The listing builds one solid part. Answer for the finished solid, in the listing's coordinates (mm). Face numbers are marked on the shaded views. A direction names the side the tool comes from. Round coordinates to 2 decimals unless told otherwise and drop trailing zeros. Write each loop counter-clockwise with the first axis right and the second up, starting at its lowest first coordinate (ties: lowest second). Pieces come first, ordered by that corner, then holes. Notation, with made-up numbers: (-2.75, 22) - (4.25, 22) arc R30 ccw to (4.25, 52) - close; hole circle Ø3 at (11.25, 66.25). An arc over 180 degrees is marked (long way). Answer in a Markdown table with one row per item.
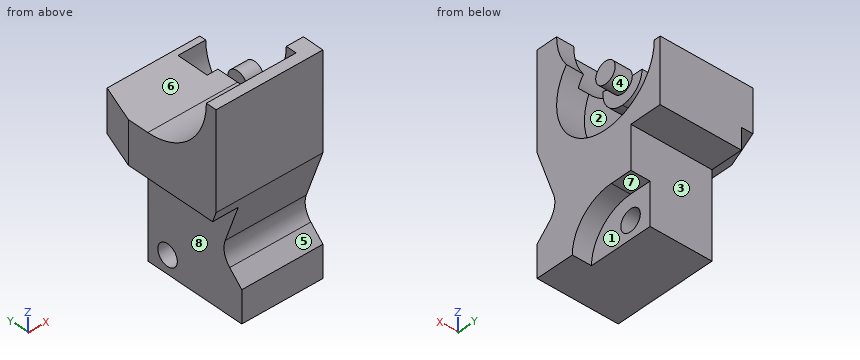
from build123d import *

# Parameters (mm, degrees)
SKETCH1_W           = 100
SKETCH1_H           = 63
BOSS_EXTRUDE1_DEPTH = 50
SKETCH2_W           = 50
SKETCH2_H           = 40
CUT_EXTRUDE1_DEPTH  = 15
SKETCH3_W           = 12
SKETCH3_H           = 10
CUT_EXTRUDE2_DEPTH  = 15
CUT_EXTRUDE3_DEPTH  = 9
SKETCH5_R           = 5
CUT_EXTRUDE4_DEPTH  = 42
CUT_EXTRUDE5_DEPTH  = 51
CUT_EXTRUDE6_DEPTH  = 42
CUT_EXTRUDE10_DEPTH = 51
CUT_EXTRUDE16_DEPTH = 13
CUT_EXTRUDE17_DEPTH = 8
SKETCH11_10_R       = 5
BOSS_EXTRUDE5_DEPTH = 8
CUT_EXTRUDE18_DEPTH = 20
CUT_EXTRUDE22_DEPTH = 8
SKETCH16_W          = 12
SKETCH16_H          = 50
CUT_EXTRUDE23_DEPTH = 49


with BuildPart() as part:
    # Sketch1 → Boss-Extrude1 (new body)
    with BuildSketch(Plane(origin=(0, 0, 0), x_dir=(0, 0, -1), z_dir=(1, 0, 0))):
        with Locations((6.649757701, 6.248490946)):
            Rectangle(SKETCH1_W, SKETCH1_H)
    extrude(amount=-BOSS_EXTRUDE1_DEPTH)

    # Sketch2 → Cut-Extrude1 (cut)
    with BuildSketch(Plane(origin=(0, 37.748490946, 0), x_dir=(1, 0, 0), z_dir=(0, 1, 0))):
        with Locations((-25, 36.649757701)):
            Rectangle(SKETCH2_W, SKETCH2_H)
    extrude(amount=-CUT_EXTRUDE1_DEPTH, mode=Mode.SUBTRACT)

    # Sketch3 → Cut-Extrude2 (cut)
    with BuildSketch(Plane(origin=(0, 37.748490946, 0), x_dir=(1, 0, 0), z_dir=(0, 1, 0))):
        with Locations((-44, 11.649757701)):
            Rectangle(SKETCH3_W, SKETCH3_H)
    extrude(amount=-CUT_EXTRUDE2_DEPTH, mode=Mode.SUBTRACT)

    # Sketch4 → Cut-Extrude3 (cut)
    with BuildSketch(Plane(origin=(0, 0, 0), x_dir=(0, 0, -1), z_dir=(1, 0, 0))):
        with BuildLine():
            Line((36.814050896, 22.748490946), (36.814050896, 12.748490946))
            ThreePointArc((36.814050896, 12.748490946), (42.613947659, -1.335438479), (56.649757701, -7.250834237))
            Line((56.649757701, -7.250834237), (56.649757701, 22.748490946))
            Line((56.649757701, 22.748490946), (36.814050896, 22.748490946))
        make_face()
    extrude(amount=-CUT_EXTRUDE3_DEPTH, mode=Mode.SUBTRACT)

    # Sketch5 → Cut-Extrude4 (cut, through all)
    with BuildSketch(Plane(origin=(-9, 0, 0), x_dir=(0, 0, -1), z_dir=(1, 0, 0))):
        with Locations((48.259112346, 12.748490946)):
            Circle(SKETCH5_R)
    extrude(amount=-CUT_EXTRUDE4_DEPTH, mode=Mode.SUBTRACT)

    # Sketch6 → Cut-Extrude5 (cut, through all)
    with BuildSketch(Plane(origin=(0, 0, 0), x_dir=(0, 0, -1), z_dir=(1, 0, 0))):
        with BuildLine():
            Line((41.649757701, -25.251509054), (35.480677879, -19.082429233))
            ThreePointArc((35.480677879, -19.082429233), (30.574006207, -16.390536973), (24.989408634, -16.756570837))
            Line((24.989408634, -16.756570837), (1.649757701, -25.251509054))
            Line((1.649757701, -25.251509054), (41.649757701, -25.251509054))
        make_face()
    extrude(amount=-CUT_EXTRUDE5_DEPTH, mode=Mode.SUBTRACT)

    # Sketch8 → Cut-Extrude6 (cut)
    with BuildSketch(Plane.ZY.offset(50)):
        with BuildLine():
            Line((43.350242299, -20.251509054), (43.350242299, 9.748490946))
            Line((43.350242299, 9.748490946), (13.350242299, 9.748490946))
            ThreePointArc((13.350242299, 9.748490946), (22.137038863, -11.46471249), (43.350242299, -20.251509054))
        make_face()
    extrude(amount=-CUT_EXTRUDE6_DEPTH, mode=Mode.SUBTRACT)

    # Sketch8<5> → Cut-Extrude10 (cut, through all)
    with BuildSketch(Plane.ZY.offset(50)):
        Polygon((13.350242299, 9.748490946), (43.350242299, 9.748490946), (43.350242299, 37.748490946), (36.798778082, 37.748490946), (13.350242299, 37.748490946), align=None)
    extrude(amount=-CUT_EXTRUDE10_DEPTH, mode=Mode.SUBTRACT)

    # Sketch11 → Cut-Extrude16 (cut)
    with BuildSketch(Plane(origin=(0, 0, 0), x_dir=(0, 0, -1), z_dir=(1, 0, 0))):
        with BuildLine():
            ThreePointArc((-23.350242299, 9.748490946), (-20.421310111, 16.819558758), (-13.350242299, 19.748490946))
            Line((-13.350242299, 19.748490946), (-13.350242299, 34.748490946))
            ThreePointArc((-13.350242299, 34.748490946), (-31.027911829, 27.426160475), (-38.350242299, 9.748490946))
            Line((-38.350242299, 9.748490946), (-23.350242299, 9.748490946))
        make_face()
        with BuildLine():
            Line((-13.350242299, 34.748490946), (-13.350242299, 19.748490946))
            ThreePointArc((-13.350242299, 19.748490946), (-6.279174487, 16.819558758), (-3.350242299, 9.748490946))
            ThreePointArc((-3.350242299, 9.748490946), (-13.350242299, -0.251509054), (-23.350242299, 9.748490946))
            Line((-23.350242299, 9.748490946), (-38.350242299, 9.748490946))
            ThreePointArc((-38.350242299, 9.748490946), (-35.710922074, -1.431848942), (-28.350242299, -10.251509054))
            ThreePointArc((-28.350242299, -10.251509054), (-2.169902411, -12.612188829), (11.649757701, 9.748490946))
            ThreePointArc((11.649757701, 9.748490946), (4.327427231, 27.426160475), (-13.350242299, 34.748490946))
        make_face()
    extrude(amount=-CUT_EXTRUDE16_DEPTH, mode=Mode.SUBTRACT)

    # Sketch11<8> → Cut-Extrude17 (cut)
    with BuildSketch(Plane(origin=(0, 0, 0), x_dir=(0, 0, -1), z_dir=(1, 0, 0))):
        with BuildLine():
            ThreePointArc((-3.350242299, 9.748490946), (-6.279174487, 16.819558758), (-13.350242299, 19.748490946))
            Line((-13.350242299, 19.748490946), (-13.350242299, 14.748490946))
            ThreePointArc((-13.350242299, 14.748490946), (-9.814708393, 13.284024852), (-8.350242299, 9.748490946))
            ThreePointArc((-8.350242299, 9.748490946), (-13.350242299, 4.748490946), (-18.350242299, 9.748490946))
            Line((-18.350242299, 9.748490946), (-23.350242299, 9.748490946))
            ThreePointArc((-23.350242299, 9.748490946), (-13.350242299, -0.251509054), (-3.350242299, 9.748490946))
        make_face()
    extrude(amount=-CUT_EXTRUDE17_DEPTH, mode=Mode.SUBTRACT)

    # Sketch11<10> → Boss-Extrude5 (add)
    with BuildSketch(Plane(origin=(0, 0, 0), x_dir=(0, 0, -1), z_dir=(1, 0, 0))):
        with Locations((-13.350242299, 9.748490946)):
            Circle(SKETCH11_10_R)
    extrude(amount=-BOSS_EXTRUDE5_DEPTH)

    # Sketch14 → Cut-Extrude18 (cut)
    with BuildSketch(Plane.XY.offset(13.350242299)):
        Polygon((-50, 19.748490946), (-43.448535783, 37.748490946), (-50, 37.748490946), align=None)
    extrude(amount=-CUT_EXTRUDE18_DEPTH, mode=Mode.SUBTRACT)

    # Sketch11<11> → Cut-Extrude22 (cut)
    with BuildSketch(Plane(origin=(0, 0, 0), x_dir=(0, 0, -1), z_dir=(1, 0, 0))):
        with BuildLine():
            ThreePointArc((-28.350242299, -10.251509054), (-35.710922074, -1.431848942), (-38.350242299, 9.748490946))
            Line((-38.350242299, 9.748490946), (-43.350242299, 9.748490946))
            Line((-43.350242299, 9.748490946), (-43.350242299, -15.251509054))
            ThreePointArc((-43.350242299, -15.251509054), (-35.444548148, -13.968591506), (-28.350242299, -10.251509054))
        make_face()
    extrude(amount=-CUT_EXTRUDE22_DEPTH, mode=Mode.SUBTRACT)

    # Sketch16 → Cut-Extrude23 (cut, through all)
    with BuildSketch(Plane(origin=(0, 22.748490946, 0), x_dir=(1, 0, 0), z_dir=(0, 1, 0))):
        with Locations((-44, 31.649757701)):
            Rectangle(SKETCH16_W, SKETCH16_H)
    extrude(amount=-CUT_EXTRUDE23_DEPTH, mode=Mode.SUBTRACT)


solid = part.part
(1) Section D-D (z = 6) is taken. Give the vertices of the cut face in (x, y).
Checked values:
| item | result |
|---|---|
| outline | (-50, -25.25) - (0, -25.25) - (0, -14.15) - (-13, -14.15) - (-13, 2.97) - (-8, 2.97) - (-8, 16.53) - (-13, 16.53) - (-13, 33.64) - (0, 33.64) - (0, 37.75) - (-43.45, 37.75) - (-50, 19.75) - close |
(2) Find the intervals of material crossed by line 1 (X direction, y = -13, z = -12.5); line 2 (Z direction, x = -17, y = 25); line 3 (X direction, y = -15, z = 32), in increasing order.
Checked values:
| item | result |
|---|---|
| line 1 | x = -38 to 0 |
| line 2 | z = -16.65 to 13.35 |
| line 3 | x = -8 to 0 |
(3) Section A-A (x = -17) is taken. Give the vertices of the cut face in (y, z), and give its area (3 significant figures).
Checked values:
| item | result |
|---|---|
| outline | (-25.25, -56.65) - (22.75, -56.65) - (22.75, -16.65) - (37.75, -16.65) - (37.75, 13.35) - (9.75, 13.35) arc R30 cw to (-20.25, 43.35) - (-25.25, 43.35) - (-25.25, -1.65) - (-16.76, -24.99) arc R10 cw to (-19.08, -35.48) - (-25.25, -41.65) - close; hole circle Ø10 at (12.75, -48.26) |
| area | 3,870 mm2 |
(4) Section C-C (z = -46.5) is taken. Give the vertices of the cut face in (x, y), and give its area (3 significant figures).
Checked values:
| item | result |
|---|---|
| outline | (-38, -25.25) - (0, -25.25) - (0, -4.39) - (-9, -4.39) - (-9, 8.07) - (-38, 8.07) - close; (-38, 17.43) - (-9, 17.43) - (-9, 22.75) - (-38, 22.75) - close |
| area | 1,310 mm2 |
(5) Flat-ended cylindrical pins translate along their axes: pin 1 (1.5 mm diameter, centred on x = -17.5, z = -11, fed in from -Y); pin 2 (11.5 mm diameter, centred on x = -24, z = -34.5, fed in from +Y); pin 3 (6 mm diameter, centred on x = -6, z = -16.5, fed in from -Y). Find the tip coordinate at first contact, or state that the pin passes through.
Checked values:
| item | result |
|---|---|
| pin 1 | stops at y = -22.12 |
| pin 2 | stops at y = 22.75 |
| pin 3 | stops at y = -20.94 |
(6) For a pull along Y with two mould halves and no side action, classify the marked faces 1, 2 and 3 as pulls with the +Y half, pulls with the -Y half, needs draft (parallel to the pull), parting line crosses it, or undercut.
Checked values:
| item | result |
|---|---|
| face 1 | needs draft |
| face 2 | undercut |
| face 3 | pulls with the +Y half |
(7) For the marked faces 4, 5, 6, 7 and 8, determine the directions among +Z, -Z, +X, -X, +Y, -Y from which every point of the face is accessible in a straight line to the end or side of a thin tool.
Checked values:
| item | result |
|---|---|
| face 4 | +X |
| face 5 | +X, -X, -Y |
| face 6 | +Z, -X, +Y |
| face 7 | -Z, +X, +Y |
| face 8 | -Z, -X, +Y, -Y |
(8) Section B-B (y = -8.5) is taken. Give the vertices of the cut face in (x, z), and give its area (3 significant figures).
Checked values:
| item | result |
|---|---|
| outline | (-50, -6.65) - (-38, -6.65) - (-38, -56.65) - (0, -56.65) - (0, -3.74) - (-13, -3.74) - (-13, 19.54) - (-50, 19.54) - close |
| area | 2,910 mm2 |
